Design review of the part built by this model. Coordinates are the model's own, in mm. A direction names the side the tool comes from. Coordinates: 2 decimals unless noted, no trailing zeros. Loops run counter-clockwise (first coordinate to the right, second up) from the corner with the lowest first, then second, coordinate; pieces in that order, holes last. Notation, with made-up numbers: (42.25, -40) -> (72.25, -40) arc R31 cw to (72.25, -2) -> close; hole circle Ø10 at (-31, -11). An arc over 180 degrees is marked (long way). Use one line per item in the form item = value. Start each with the question number.
1. Machinability: for faces 1 (the face through (-18.8, -1.25, 8.7)), 2 (the face through (18, -1, 3)), 3 (the face through (-19.1, -1, 7)), 4 (the face through (19, 0, 7.9)), 5 (the face through (19, 10, 10)), which of the approach directions +Z, -Z, +X, -X, +Y, -Y give a long, thin tool a straight path to every point of the face, cutting with its end or side? Answer none if there is none.
2. The part is to be moulded in two halves that separate along Y. For faces 6 (the face through (0, -31, 1)), 7 (the face through (18, -7, 9)), 8 (the face through (18.8, -1.25, 8.7)), say which applies: released by +Y, released by -Y, zero draft, split by the parting line, or undercut.
3. Consider section B-B (y = 11). State the section outline as (x, z) points, then the cut area to 3 significant figures.
4. Consider section A-A (z = 6.5). State the section outline as (x, y) points.
5. Consider section C-C (x = -12). State the section outline as (y, z) points, then the cut area to 3 significant figures.
6. Wall thickness on line 1 (X direction, y = 4, z = 8); line 2 (X direction, y = -25.5, z = 6); line 3 (Y direction, x = 13.5, z = 6.25): over which ranges is each line inside the solid? List them lowest first. Write a range as from..to.
7. For pin 1 (1.1 mm diameter, centred on y = -30.5, z = 0.5, fed in from +X); pin 2 (2 mm diameter, centred on x = 18.5, z = 6, fed in from -Y); pin 3 (2 mm diameter, centred on x = -15, y = 22.5, fed in from +Z); pin 4 (6 mm diameter, centred on x = 7.5, z = 9, fed in from -Y), all flat-tipped, find the tip position at first contact; note any pin that passes through.
from build123d import *

# Parameters (mm, degrees)
SKETCH_1_W          = 40
SKETCH_1_H          = 62
EXTRUDE_1_DEPTH     = 10
SKETCH_2_W          = 36
SKETCH_2_H          = 58
CUT_EXTRUDE_1_DEPTH = 8.5
SKETCH_4_W          = 36
SKETCH_4_H          = 8.5
CUT_EXTRUDE_2_DEPTH = 2
SKETCH_5_W          = 38.2
SKETCH_5_H          = 2.1
CUT_EXTRUDE_3_DEPTH = 60
SKETCH_6_W          = 40
SKETCH_6_H          = 10
CUT_EXTRUDE_4_DEPTH = 1
SKETCH_7_W          = 38.4
SKETCH_7_H          = 1.5
EXTRUDE_2_DEPTH     = 1
SKETCH_8_W          = 1.2
SKETCH_8_H          = 2.7
CUT_EXTRUDE_5_DEPTH = 52.584881506
SKETCH_10_W         = 0.9
SKETCH_10_H         = 2.7
CUT_EXTRUDE_6_DEPTH = 1


with BuildPart() as part:
    # 草图1 → 凸台-拉伸1 (new body)
    with BuildSketch(Plane.XY):
        Rectangle(SKETCH_1_W, SKETCH_1_H)
    extrude(amount=EXTRUDE_1_DEPTH)

    # 草图2 → 切除-拉伸1 (cut)
    with BuildSketch(Plane.XY.offset(10)):
        Rectangle(SKETCH_2_W, SKETCH_2_H)
    extrude(amount=-CUT_EXTRUDE_1_DEPTH, mode=Mode.SUBTRACT)

    # 草图4 → 切除-拉伸2 (cut)
    with BuildSketch(Plane.XZ.offset(31)):
        with Locations((0, 5.75)):
            Rectangle(SKETCH_4_W, SKETCH_4_H)
    extrude(amount=-CUT_EXTRUDE_2_DEPTH, mode=Mode.SUBTRACT)

    # 草图5 → 切除-拉伸3 (cut)
    with BuildSketch(Plane.XZ.offset(31)):
        with Locations((0, 6.55)):
            Rectangle(SKETCH_5_W, SKETCH_5_H)
    extrude(amount=-CUT_EXTRUDE_3_DEPTH, mode=Mode.SUBTRACT)

    # 草图6 → 切除-拉伸4 (cut)
    with BuildSketch(Plane.XZ.offset(31)):
        with Locations((0, 5)):
            Rectangle(SKETCH_6_W, SKETCH_6_H)
    extrude(amount=-CUT_EXTRUDE_4_DEPTH, mode=Mode.SUBTRACT)

    # 草图7 → 凸台-拉伸2 (add)
    with BuildSketch(Plane.XZ.offset(30)):
        with Locations((-0.2, 0.75)):
            Rectangle(SKETCH_7_W, SKETCH_7_H)
    extrude(amount=EXTRUDE_2_DEPTH)

    # 草图8 → 切除-拉伸5 (cut, through all)
    with BuildSketch(Plane.ZY.offset(20)):
        with Locations((8.5, 0.1)):
            Rectangle(SKETCH_8_W, SKETCH_8_H)
    extrude(amount=-CUT_EXTRUDE_5_DEPTH, mode=Mode.SUBTRACT)

    # 草图10 → 切除-拉伸6 (cut)
    with BuildSketch(Plane(origin=(-18, 0, 0), x_dir=(0, 0, -1), z_dir=(1, 0, 0))):
        with Locations((-9.55, 0.1)):
            Rectangle(SKETCH_10_W, SKETCH_10_H)
    cut_extrude_6 = extrude(amount=-CUT_EXTRUDE_6_DEPTH, mode=Mode.SUBTRACT)

    # 镜向1: 切除-拉伸6 across plane
    add(cut_extrude_6.mirror(Plane(origin=(0, 0, 0), x_dir=(0, 0, 1), z_dir=(1, 0, 0))), mode=Mode.SUBTRACT)


solid = part.part
Geometry check:
q1.face_1 = none
q1.face_2 = +Z, -Y
q1.face_3 = -Y
q1.face_4 = +X, -X
q1.face_5 = +Z, +X, -X, +Y, -Y
q2.face_6 = released by -Y
q2.face_7 = zero draft
q2.face_8 = undercut
q3.outline = (-20, 0) -> (20, 0) -> (20, 10) -> (18, 10) -> (18, 7.6) -> (19.1, 7.6) -> (19.1, 5.5) -> (18, 5.5) -> (18, 1.5) -> (-18, 1.5) -> (-18, 5.5) -> (-19.1, 5.5) -> (-19.1, 7.6) -> (-18, 7.6) -> (-18, 10) -> (-20, 10) -> close
q3.area = 89.4 mm²
q4.outline = (-20, -30) -> (-19.1, -30) -> (-19.1, 29) -> (19.1, 29) -> (19.1, -30) -> (20, -30) -> (20, 31) -> (-20, 31) -> close
q5.outline = (-31, 0) -> (31, 0) -> (31, 10) -> (29, 10) -> (29, 1.5) -> (-31, 1.5) -> close
q5.area = 110 mm²
q6.line_1 = -20..-18, 18..20
q6.line_2 = -20..-19.1, 19.1..20
q6.line_3 = 29..31
q7.pin_1 = 20
q7.pin_2 = -30
q7.pin_3 = 1.5
q7.pin_4 = 29
